```python
from build123d import *

# Parameters (mm, degrees)
SKETCH_2_R      = 1.5
SKETCH_2_R_2    = 1
EXTRUDE_1_DEPTH = 4
FILLET_1_R      = 7


with BuildPart() as part:
    # 草圖2 → 填料-伸長1 (new body)
    with BuildSketch(Plane(origin=(0, 0, 0), x_dir=(-1, 0, 0), z_dir=(0, 1, 0))):
        Polygon((32.696699141, -32.696699141), (-32.696699141, -32.696699141), (-44.696699141, -32.696699141), (-44.696699141, -20.696699141), (-44.696699141, 20.696699141), (-44.696699141, 32.696699141), (-32.696699141, 32.696699141), (32.696699141, 32.696699141), (44.696699141, 32.696699141), (44.696699141, 20.696699141), (44.696699141, -20.696699141), (44.696699141, -32.696699141), align=None)
        with Locations((38, 26)):
            Circle(SKETCH_2_R, mode=Mode.SUBTRACT)
        with Locations((38, -26)):
            Circle(SKETCH_2_R, mode=Mode.SUBTRACT)
        with Locations((-38, 26)):
            Circle(SKETCH_2_R, mode=Mode.SUBTRACT)
        with Locations((-38, -26)):
            Circle(SKETCH_2_R, mode=Mode.SUBTRACT)
        with Locations((5.700000775, -24.699999821)):
            Circle(SKETCH_2_R_2, mode=Mode.SUBTRACT)
        with Locations((-5.699999225, 24.700000179)):
            Circle(SKETCH_2_R_2, mode=Mode.SUBTRACT)
        with BuildLine():
            Line((32.696699141, -23.696699141), (11.942354682, -23.696699141))
            ThreePointArc((11.942354682, -23.696699141), (10.211256961, -23.302708109), (8.821177729, -22.198349481))
            ThreePointArc((8.821177729, -22.198349481), (5.700000775, -20.699999821), (2.578823821, -22.198349481))
            ThreePointArc((2.578823821, -22.198349481), (1.188744589, -23.302708109), (-0.542353133, -23.696699141))
            Line((-0.542353133, -23.696699141), (-32.696699141, -23.696699141))
            ThreePointArc((-32.696699141, -23.696699141), (-34.818019485, -22.818019485), (-35.696699141, -20.696699141))
            Line((-35.696699141, -20.696699141), (-35.696699141, 20.696699141))
            ThreePointArc((-35.696699141, 20.696699141), (-34.818019485, 22.818019485), (-32.696699141, 23.696699141))
            Line((-32.696699141, 23.696699141), (-11.942352846, 23.696699141))
            ThreePointArc((-11.942352846, 23.696699141), (-10.211255228, 23.302708159), (-8.821176036, 22.19834966))
            ThreePointArc((-8.821176036, 22.19834966), (-5.699999225, 20.700000179), (-2.578822415, 22.19834966))
            ThreePointArc((-2.578822415, 22.19834966), (-1.188743222, 23.302708159), (0.542354396, 23.696699141))
            Line((0.542354396, 23.696699141), (32.696699141, 23.696699141))
            ThreePointArc((32.696699141, 23.696699141), (34.818019485, 22.818019485), (35.696699141, 20.696699141))
            Line((35.696699141, 20.696699141), (35.696699141, -20.696699141))
            ThreePointArc((35.696699141, -20.696699141), (34.818019485, -22.818019485), (32.696699141, -23.696699141))
        make_face(mode=Mode.SUBTRACT)
    extrude(amount=EXTRUDE_1_DEPTH)

    # 圓角1
    fillet_1_edges = [part.edges().sort_by_distance(p)[0] for p in [
        (44.696699141, 2, -32.696699141),
        (44.696699141, 2, 32.696699141),
        (-44.696699141, 2, 32.696699141),
        (-44.696699141, 2, -32.696699141),
    ]]
    fillet(fillet_1_edges, radius=FILLET_1_R)


solid = part.part
```
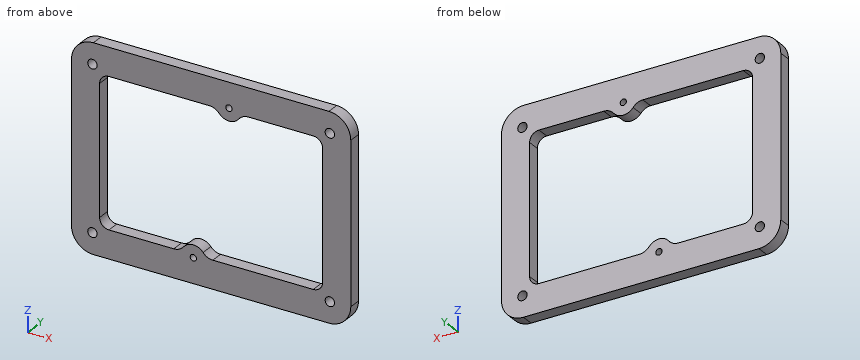
Work out the finished part from the listing and answer in its coordinate system (mm). Round coordinates to 2 decimals unless told otherwise and drop trailing zeros. Write each loop counter-clockwise with the first axis right and the second up, starting at its lowest first coordinate (ties: lowest second). Pieces come first, ordered by that corner, then holes.
1) A cutting plane is placed at D-D on x = 5.7. Determine the outline of the cut face in (y, z).
2) A cutting plane is placed at B-B on y = 3.2. Give the number of separate pieces and of enclosed holes in the cut face, and give its area (3 significant figures).
3) A cutting plane is placed at A-A on x = 22. Determine the outline of the cut face in (y, z), and give its area (3 significant figures).
4) Consider probe 1 along Z at (x, y) = (-38, 2.25); probe 2 along Z at (x, y) = (-5.7, 2.25); probe 3 along Z at (x, y) = (-25.5, 0.75). Determine where each line is inside the solid, lowest interval first.
5) A cutting plane is placed at C-C on z = -1. Determine the outline of the cut face in (x, y), and give its area (3 significant figures).
6) Flat-ended cylindrical pins translate along their axes: P1, Ø1.8, axis at x = 38, z = -26, coming from the -Y side; P2, Ø3.5, axis at x = 38, z = 26, coming from the -Y side. Find the tip coordinate at first contact, or state that the pin passes through.
Entries:
1. outline: (0, -32.7) - (4, -32.7) - (4, -23.7) - (0, -23.7) - close; (0, 20.7) - (4, 20.7) - (4, 23.7) - (0, 23.7) - close; (0, 25.7) - (4, 25.7) - (4, 32.7) - (0, 32.7) - close
2. separate pieces: 1
2. enclosed holes: 7
2. area: 2,430 mm2
3. outline: (0, -32.7) - (4, -32.7) - (4, -23.7) - (0, -23.7) - close; (0, 23.7) - (4, 23.7) - (4, 32.7) - (0, 32.7) - close
3. area: 72.0 mm2
4. probe 1: z = -32.69 to -27.5, -24.5 to 24.5, 27.5 to 32.69
4. probe 2: z = -32.7 to -25.7, -23.7 to -20.7, 23.7 to 32.7
4. probe 3: z = -32.7 to -23.7, 23.7 to 32.7
5. outline: (-44.7, 0) - (-35.7, 0) - (-35.7, 4) - (-44.7, 4) - close; (35.7, 0) - (44.7, 0) - (44.7, 4) - (35.7, 4) - close
5. area: 72.0 mm2
6. P1: passes through
6. P2: stops at y = 0
